from build123d import *

# Parameters (mm, degrees)
SKETCH_1_R               = 27.5
EXTRUDE_1_DEPTH          = 2
SKETCH_2_R               = 17.5
EXTRUDE_4_DEPTH          = 28
EXTRUDE_START            = -2
SKETCH_4_R               = 27.5
EXTRUDE_5_DEPTH          = 2
SHELL_1_OUTLINE_R        = 15.5
SHELL_1_DEPTH            = 28
SKETCH_5_R               = 27.5
SKETCH_5_R_2             = 10
EXTRUDE_6_DEPTH          = 2
SKETCH_6_R               = 12
SKETCH_6_R_2             = 10
EXTRUDE_7_DEPTH          = 26
RIB_START                = -0.5
RIB_1_OUTLINE_W          = 7
RIB_1_OUTLINE_H          = 25.5
RIB_1_DEPTH              = 1
PATTERN_CIRCULAR_1_COUNT = 4
SKETCH_9_R               = 15.5
SKETCH_9_R_2             = 15.3
EXTRUDE_8_DEPTH          = 25.5
CUT_EXTRUDE_2_DEPTH      = 48.921811318
CUT_EXTRUDE_START        = -0.2
SKETCH_10_R              = 25.5
SKETCH_10_R_2            = 17.5
CUT_EXTRUDE_3_DEPTH      = 0.2


# Read off the part's stored shape, not the designer's step: 抽壳1, 筋1
with BuildPart() as part:
    # 草图1 → 凸台-拉伸1 (new body)
    with BuildSketch(Plane(origin=(0, 0, 0), x_dir=(1, 0, 0), z_dir=(0, 1, 0))):
        with Locations(Location((0, 0, 0), (0, 0, 270))):
            Circle(SKETCH_1_R)
    extrude(amount=EXTRUDE_1_DEPTH)

    # 草图2 → 凸台-拉伸4 (add)
    with BuildSketch(Plane.XZ):
        with Locations(Location((0, 0, 0), (0, 0, 270))):
            Circle(SKETCH_2_R)
    extrude(amount=-EXTRUDE_4_DEPTH)

    # 草图4 → 凸台-拉伸5 (add)
    with BuildSketch(Plane(origin=(0, 28, 0), x_dir=(1, 0, 0), z_dir=(0, 1, 0)).offset(EXTRUDE_START)):
        with Locations(Location((0, 0, 0), (0, 0, 270))):
            Circle(SKETCH_4_R)
    extrude(amount=EXTRUDE_5_DEPTH)

    # 抽壳1 outline → 抽壳1 (cut)
    with BuildSketch(Plane(origin=(0, 0, 0), x_dir=(1, 0, 0), z_dir=(0, 1, 0))):
        Circle(SHELL_1_OUTLINE_R)
    extrude(amount=SHELL_1_DEPTH, mode=Mode.SUBTRACT)

    # 草图5 → 凸台-拉伸6 (add)
    with BuildSketch(Plane.XZ):
        with Locations(Location((0, 0, 0), (0, 0, 90))):
            Circle(SKETCH_5_R)
        with Locations(Location((0, 0, 0), (0, 0, 270))):
            Circle(SKETCH_5_R_2, mode=Mode.SUBTRACT)
    extrude(amount=-EXTRUDE_6_DEPTH)

    # 草图6 → 凸台-拉伸7 (add)
    with BuildSketch(Plane(origin=(0, 2, 0), x_dir=(1, 0, 0), z_dir=(0, 1, 0))):
        with Locations(Location((0, 0, 0), (0, 0, 90))):
            Circle(SKETCH_6_R)
        with Locations(Location((0, 0, 0), (0, 0, 90))):
            Circle(SKETCH_6_R_2, mode=Mode.SUBTRACT)
    extrude(amount=EXTRUDE_7_DEPTH)

    # 筋1 outline → 筋1 (add)
    with BuildSketch(Plane.XY.offset(RIB_START)):
        with Locations((13.5, 14.75)):
            Rectangle(RIB_1_OUTLINE_W, RIB_1_OUTLINE_H)
    rib_1 = extrude(amount=RIB_1_DEPTH)

    # 阵列(圆周)1: 筋1 ×4 about axis
    pattern_circular_1_axis = Axis((0, 0, 0), (0, 1, 0))
    for i in range(1, PATTERN_CIRCULAR_1_COUNT):
        add(rib_1.rotate(pattern_circular_1_axis, i * 360 / PATTERN_CIRCULAR_1_COUNT))

    # 草图9 → 凸台-拉伸8 (add)
    with BuildSketch(Plane(origin=(0, 2, 0), x_dir=(1, 0, 0), z_dir=(0, 1, 0))):
        with Locations(Location((0, 0, 0), (0, 0, 90))):
            Circle(SKETCH_9_R)
        Circle(SKETCH_9_R_2, mode=Mode.SUBTRACT)
    extrude(amount=EXTRUDE_8_DEPTH)

    # 草图8 → 切除-拉伸2 (cut, through all)
    with BuildSketch(Plane(origin=(0, 0, 0), x_dir=(0, 1, 0), z_dir=(0.7071067811865488, 0, 0.7071067811865464))):
        Polygon((26, 2), (26, -2), (22, 0), align=None)
    cut_extrude_2 = extrude(amount=-CUT_EXTRUDE_2_DEPTH, mode=Mode.SUBTRACT)

    # 镜向2: 切除-拉伸2 across plane
    add(cut_extrude_2.mirror(Plane.ZX.offset(14)), mode=Mode.SUBTRACT)

    # 草图10 → 切除-拉伸3 (cut)
    with BuildSketch(Plane(origin=(0, 28, 0), x_dir=(1, 0, 0), z_dir=(0, 1, 0)).offset(CUT_EXTRUDE_START)):
        with Locations(Location((0, 0, 0), (0, 0, 270))):
            Circle(SKETCH_10_R)
        with Locations(Location((0, 0, 0), (0, 0, 128.437572131))):
            Circle(SKETCH_10_R_2, mode=Mode.SUBTRACT)
    cut_extrude_3 = extrude(amount=CUT_EXTRUDE_3_DEPTH, mode=Mode.SUBTRACT)

    # 镜向3: 切除-拉伸3 across plane
    add(cut_extrude_3.mirror(Plane.ZX.offset(14)), mode=Mode.SUBTRACT)


solid = part.part
Could you check a few things on this model? Use its own coordinates, in mm. A direction names the side the tool comes from. Give positions to 0.01 mm unless a question says otherwise; leave off trailing zeros. Order: outer loops, then holes, each group sorted by start corner. A loop starts at its lowest first (then second) coordinate and runs counter-clockwise, first axis right, second up.
1. Suppose I cut it at B-B (z = 19). Write out the boundary of the cut face in (x, y).
Answers below:
outline: (-19.88, 0) - (-17.01, 0) - (-17.01, 0.2) - (17.01, 0.2) - (17.01, 0) - (19.88, 0) - (19.88, 2) - (-19.88, 2) - close; (-19.88, 26) - (19.88, 26) - (19.88, 28) - (17.01, 28) - (17.01, 27.8) - (-17.01, 27.8) - (-17.01, 28) - (-19.88, 28) - close
2. Thinking about a two-plate mould opening in Y: for faces 1 (the flat face through (-12.236, 23.972, -10.841)), 2 (the flat face through (-8, 26, -8)), 3 (the flat face through (-0.5, 15, 14)), 4 (the flat face through (-9, 28, 5)), which applies, +Y half, -Y half, draft (parallel to the pull), parting line (faces both ways), or undercut?
Answers below:
face 1: undercut
face 2: undercut
face 3: draft
face 4: +Y half
3. For pin 1 (8 mm diameter, centred on x = -12.5, y = 3.5, fed in from +Z); pin 2 (1.7 mm diameter, centred on y = 10.5, z = 14.5, fed in from +X); pin 3 (1 mm diameter, centred on y = 3.5, z = -1, fed in from +X), each with a flat end and sliding along its axis, tell me the tip position at first contact or that it passes through.
Answers below:
pin 1: stops at z = 26.06
pin 2: stops at x = 10.95
pin 3: stops at x = 17.49
4. Suppose I cut it at C-C (x = -23.5). Write out the boundary of the cut face in (y, z), plus the area to 3 significant figures.
Answers below:
outline: (0, -14.28) - (2, -14.28) - (2, 14.28) - (0, 14.28) - (0, 9.9) - (0.2, 9.9) - (0.2, -9.9) - (0, -9.9) - close; (26, -14.28) - (28, -14.28) - (28, -9.9) - (27.8, -9.9) - (27.8, 9.9) - (28, 9.9) - (28, 14.28) - (26, 14.28) - close
area: 106 mm2
5. I need wall thicknesses on L1, parallel to X at y = 27.95, z = 0; L2, parallel to X at y = 10, z = 7.5; L3, parallel to Y at x = -22, z = -1.5. Which ranges of each line are inside material? Lowest first, please.
Answers below:
L1: x = -27.5 to -25.5, -17.5 to -15.5, -12 to -10, 10 to 12, 15.5 to 17.5, 25.5 to 27.5
L2: x = -15.81 to -13.34, -9.37 to -6.61, 6.61 to 9.37, 13.34 to 15.81
L3: y = 0.2 to 2, 26 to 27.8
6. Suppose I cut it at D-D (y = 2.75). Write out the boundary of the cut face in (x, z).
Answers below:
outline: (-15.29, -0.5) - (-11.99, -0.5) arc R12 ccw to (-9.56, -7.26) - (-8.13, -5.83) arc R10 cw (long way) to (-5.83, -8.13) - (-7.26, -9.56) arc R12 ccw to (-0.5, -11.99) - (-0.5, -15.29) arc R15.3 cw to (-9.61, -11.91) - (-11.17, -13.47) arc R17.5 ccw (long way) to (-13.47, -11.17) - (-11.91, -9.61) arc R15.3 cw to start; hole (-15.29, 0.5) - (-11.99, 0.5) arc R12 cw to (-0.5, 11.99) - (-0.5, 15.29) arc R15.3 ccw to start; hole (0.5, -15.29) arc R15.3 ccw to (15.29, -0.5) - (11.99, -0.5) arc R12 cw to (0.5, -11.99) - close; hole (0.5, 11.99) arc R12 cw to (11.99, 0.5) - (15.29, 0.5) arc R15.3 ccw to (0.5, 15.29) - close
7. Which directions (+Z, -Z, +X, -X, +Y, -Y) give clear straight access to the entire face, cutting with the end or side of a thin tool? Please do faces 5 (the cylindrical face through (-2.018, 27.746, -15.368)), 6 (the flat face through (-8.39, 23.97, -7)), 7 (the flat face through (-18.2, 28, 18.2)).
Answers below:
face 5: +Y
face 6: none
face 7: +Z, -Z, +X, -X, +Y
8. Suppose I cut it at A-A (y = 16). Write out the boundary of the cut face in (x, z), plus the area to 3 significant figures.
Answers below:
outline: circle Ø35 at (0, 0); hole (-15.29, -0.5) arc R15.3 ccw to (-0.5, -15.29) - (-0.5, -11.99) arc R12 cw to (-11.99, -0.5) - close; hole (-15.29, 0.5) - (-11.99, 0.5) arc R12 cw to (-0.5, 11.99) - (-0.5, 15.29) arc R15.3 ccw to start; hole circle Ø20 at (0, 0); hole (0.5, -15.29) arc R15.3 ccw to (15.29, -0.5) - (11.99, -0.5) arc R12 cw to (0.5, -11.99) - close; hole (0.5, 11.99) arc R12 cw to (11.99, 0.5) - (15.29, 0.5) arc R15.3 ccw to (0.5, 15.29) - close
area: 378 mm2
